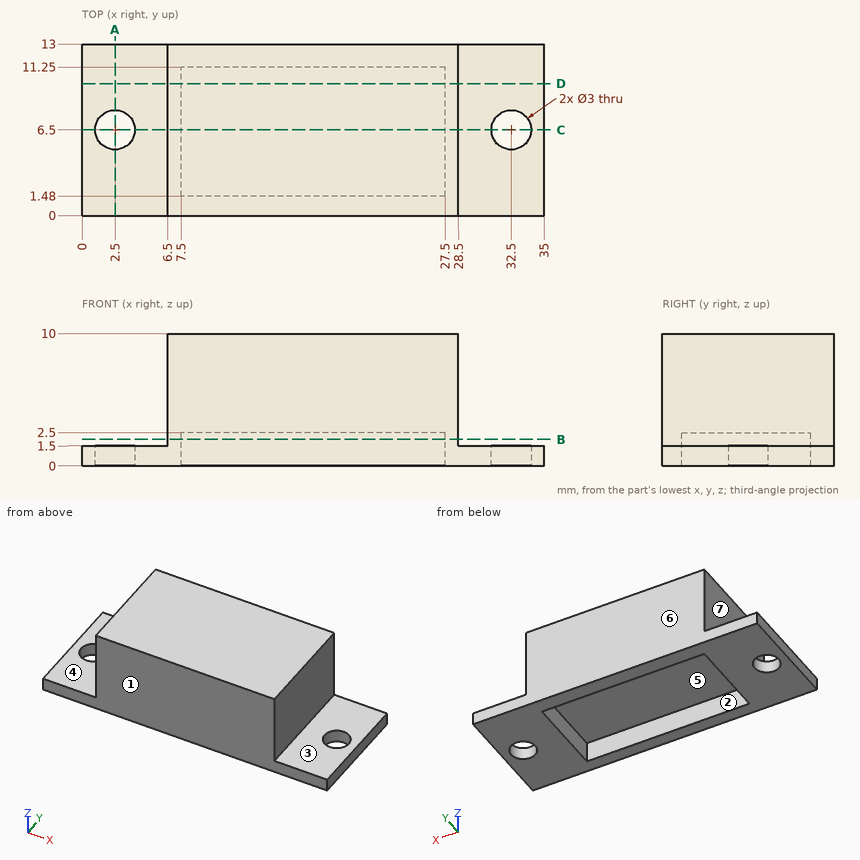
Can you work these out from the drawing? Everything is in mm from the part's minimum corner. A direction names the side the tool comes from. Give positions to 0.01 mm unless a question says otherwise; leave off trailing zeros. Write each loop counter-clockwise with the first axis right and the second up, starting at its lowest first coordinate (ties: lowest second). Pieces come first, ordered by that corner, then holes. Notation, with made-up numbers: M 55.25,7.5 L 77.25,7.5 A22 cw 77.25,24.5 Z; hole C 68.25,6.5 d1. An arc over 180 degrees is marked long. Answer in a Markdown table with one row per item. Add a question column.
Item 1: For pin 1 Ø2.5 at (x, y) = (32.5, 6.5) entering from +Z; pin 2 Ø1.5 at (x, y) = (18, 7) entering from -Z; pin 3 Ø2 at (x, z) = (21, 1.5) entering from -Y; pin 4 Ø3 at (x, y) = (4, 3.5) entering from +Z, each with a flat end and sliding along its axis, tell me the tip position at first contact or that it passes through.
Item 2: Please list where these lines run through material, in increasing order: L1, parallel to Y at x = 2.5, z = 0.8; L2, parallel to Z at x = 14, y = 9; L3, parallel to X at y = 10.5, z = 8.5.
Item 3: We'd pull the mould along X, two halves only. Please class the marked faces 5, 6 and 7: released by +X, released by -X, zero draft, split by the parting line, or undercut.
Item 4: On a 3-axis mill with a long thin cutter (end or side, diameter ignored), from which of +Z, -Z, +X, -X, +Y, -Y can I reach the whole of each face in a straight line? I mean the marked faces 1, 2, 3 and 4. Say none if no direction works.
Item 5: Imagine slicing it at B-B, the plane z = 2. Write out the boundary of the cut face in (x, y).
Item 6: Imagine slicing it at D-D, the plane y = 10. Write out the boundary of the cut face in (x, z).
Item 7: Imagine slicing it at A-A, the plane x = 2.5. Write out the boundary of the cut face in (y, z), plus the area to 3 significant figures.
Item 8: Imagine slicing it at C-C, the plane y = 6.5. Write out the boundary of the cut face in (x, z).
Evaluation:
| question | item | result |
|---|---|---|
| 1 | pin 1 | passes through |
| 1 | pin 2 | stops at z = 2.5 |
| 1 | pin 3 | stops at y = 0 |
| 1 | pin 4 | stops at z = 1.5 |
| 2 | L1 | y = 0 to 5, 8 to 13 |
| 2 | L2 | z = 2.5 to 10 |
| 2 | L3 | x = 6.5 to 28.5 |
| 3 | face 5 | undercut |
| 3 | face 6 | zero draft |
| 3 | face 7 | released by -X |
| 4 | face 1 | +Z, -Z, +X, -X, -Y |
| 4 | face 2 | -Z |
| 4 | face 3 | +Z, +X, +Y, -Y |
| 4 | face 4 | +Z, -X, +Y, -Y |
| 5 | outline | M 6.5,0 L 28.5,0 L 28.5,13 L 6.5,13 Z; hole M 7.5,1.48 L 27.5,1.48 L 27.5,11.25 L 7.5,11.25 Z |
| 6 | outline | M 0,0 L 7.5,0 L 7.5,2.5 L 27.5,2.5 L 27.5,0 L 35,0 L 35,1.5 L 28.5,1.5 L 28.5,10 L 6.5,10 L 6.5,1.5 L 0,1.5 Z |
| 7 | outline | M 0,0 L 5,0 L 5,1.5 L 0,1.5 Z; M 8,0 L 13,0 L 13,1.5 L 8,1.5 Z |
| 7 | area | 15.0 mm² |
| 8 | outline | M 0,0 L 1,0 L 1,1.5 L 0,1.5 Z; M 4,0 L 7.5,0 L 7.5,2.5 L 27.5,2.5 L 27.5,0 L 31,0 L 31,1.5 L 28.5,1.5 L 28.5,10 L 6.5,10 L 6.5,1.5 L 4,1.5 Z; M 34,0 L 35,0 L 35,1.5 L 34,1.5 Z |
